Input: part model. Units: mm. Frame: model coordinates. Face numbers are marked on the shaded views. A direction names the side the tool comes from. Round coordinates to 2 decimals unless told otherwise and drop trailing zeros. Loops run counter-clockwise (first coordinate to the right, second up) from the corner with the lowest first, then second, coordinate; pieces in that order, holes last. Notation, with made-up numbers: (25, 62.25) -> (51, 62.25) arc R33 ccw to (51, 95.25) -> close; hole circle Ø10 at (19.5, 38). An arc over 180 degrees is marked (long way). Answer in a Markdown table with one row per item. Add a question column.
Q1. Section C-C, the plane x = -8. Output: boundary loops of the cut face in (y, z).
Q2. Section B-B, the plane y = -6. Output: boundary loops of the cut face in (x, z), and give its area (3 significant figures).
Q3. Mould query, pull axis X, two halves, no side actions, for the marked faces 3, 4, 5 and 6. Classes: pulls with the +X half, pulls with the -X half, needs draft (parallel to the pull), parting line crosses it, or undercut.
Q4. Reachability of the marked faces 1 and 2 from +Z, -Z, +X, -X, +Y, -Y: full face, straight path, thin tool, end or side. Return the list, or none.
Q5. Pin query (flat end, axial travel): pin 1 (4 mm diameter, centred on x = -11, y = 13, fed in from -Z); pin 2 (2 mm diameter, centred on x = -9, y = 17, fed in from +Z); pin 3 (4 mm diameter, centred on x = 13.5, z = 52, fed in from +Y); pin 4 (19 mm diameter, centred on x = 7.5, y = -8.5, fed in from +Z). Return the tip coordinate at first contact, or that it passes through.
Q6. Ray query, L1, parallel to Z at x = 0, y = -2; L2, parallel to Z at x = -7.5, y = -19; L3, parallel to Y at x = 14, z = 19. Return the intervals inside material, ascending. Write a range as from..to.
Q7. Section D-D, the plane y = 21. Output: boundary loops of the cut face in (x, z), and give its area (3 significant figures).
Q8. Section A-A, the plane z = -1. Output: boundary loops of the cut face in (x, y), and give its area (3 significant figures).
```python
from build123d import *

# Parameters (mm, degrees)
F0_R     = 17.5
F0_R_2   = 12.5
F1_DEPTH = 25
F2_W     = 35
F2_H     = 35
F3_DEPTH = 22.5
F4_R     = 12.5
F5_DEPTH = 50
F6_DEPTH = 35


with BuildPart() as f1:
    # F0 (on Front) → F1 (new body, symmetric)
    with BuildSketch(Plane.XZ):
        Circle(F0_R)
        Circle(F0_R_2, mode=Mode.SUBTRACT)
    extrude(amount=F1_DEPTH, both=True)

    # F2 (on Top) → F3 (join)
    with BuildSketch(Plane.XY):
        Rectangle(F2_W, F2_H)
    extrude(amount=F3_DEPTH)

    # F4 (on face) → F5 (join)
    with BuildSketch(Plane.XY.offset(22.5)):
        with BuildLine():
            ThreePointArc((3.33e-08, -17.5), (12.3743686825, -12.374368659), (17.5, 0))
            ThreePointArc((17.5, 0), (12.3743686917, 12.3743686498), (5.93e-08, 17.5))
            ThreePointArc((5.93e-08, 17.5), (-12.3743686571, 12.3743686844), (-17.5, -2.06e-08))
            ThreePointArc((-17.5, -2.06e-08), (-12.3743686517, -12.3743686898), (3.33e-08, -17.5))
        make_face()
        Circle(F4_R, mode=Mode.SUBTRACT)
    extrude(amount=F5_DEPTH)

    # F6 (cut, through all): a face of the model
    f6_faces = [f1.faces().sort_by_distance(p)[0] for p in [
        (0, -17.5, 5.3051647697),
    ]]
    extrude(f6_faces, amount=-F6_DEPTH, mode=Mode.SUBTRACT)


solid = f1.part
```
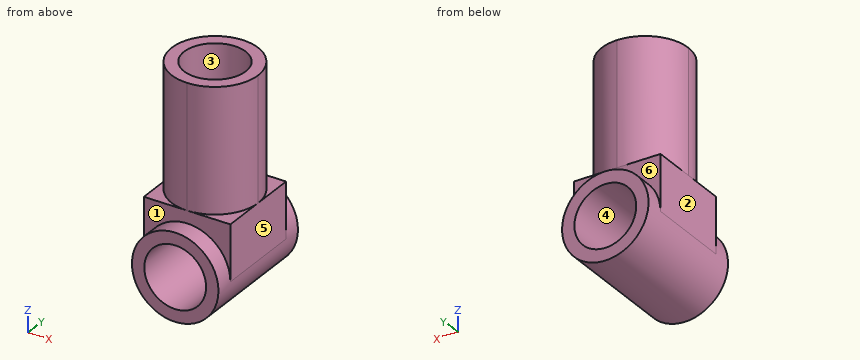
Answer block:
| question | item | result |
|---|---|---|
| 1 | outline | (-25, -15.56) -> (25, -15.56) -> (25, -9.6) -> (-25, -9.6) -> close; (-25, 9.6) -> (25, 9.6) -> (25, 15.56) -> (17.5, 15.56) -> (17.5, 22.5) -> (15.56, 22.5) -> (15.56, 72.5) -> (9.6, 72.5) -> (9.6, 22.5) -> (-9.6, 22.5) -> (-9.6, 72.5) -> (-15.56, 72.5) -> (-15.56, 22.5) -> (-17.5, 22.5) -> (-17.5, 15.56) -> (-25, 15.56) -> close |
| 2 | outline | (-17.5, 0) arc R17.5 ccw to (17.5, 0) -> (17.5, 22.5) -> (16.44, 22.5) -> (16.44, 72.5) -> (10.97, 72.5) -> (10.97, 22.5) -> (-10.97, 22.5) -> (-10.97, 72.5) -> (-16.44, 72.5) -> (-16.44, 22.5) -> (-17.5, 22.5) -> close; hole circle Ø25 at (0, 0) |
| 2 | area | 1,330 mm^2 |
| 3 | face 3 | undercut |
| 3 | face 4 | undercut |
| 3 | face 5 | pulls with the +X half |
| 3 | face 6 | needs draft |
| 4 | face 1 | +Z, -Y |
| 4 | face 2 | +Z, -Z, -X, +Y, -Y |
| 5 | pin 1 | z = -15.01 |
| 5 | pin 2 | z = 22.5 |
| 5 | pin 3 | y = 13.19 |
| 5 | pin 4 | z = 72.5 |
| 6 | L1 | -17.5..-12.5, 12.5..22.5 |
| 6 | L2 | -15.81..-10, 10..15.81 |
| 6 | L3 | -17.5..17.5 |
| 7 | outline | circle Ø35 at (0, 0); hole circle Ø25 at (0, 0) |
| 7 | area | 471 mm^2 |
| 8 | outline | (-17.47, -25) -> (-12.46, -25) -> (-12.46, 25) -> (-17.47, 25) -> close; (12.46, -25) -> (17.47, -25) -> (17.47, 25) -> (12.46, 25) -> close |
| 8 | area | 501 mm^2 |
